Part print with two shaded views. Sizes in mm from the minimum x, y, z corner. Round coordinates to 2 decimals unless told otherwise and drop trailing zeros. Write each loop counter-clockwise with the first axis right and the second up, starting at its lowest first coordinate (ties: lowest second). Pieces come first, ordered by that corner, then holes. Notation, with made-up numbers: M -22.75,13.25 L -6.75,13.25 A10 ccw -6.75,31.25 Z; hole C 85.25,75 d1. An arc over 180 degrees is marked long. One line per question, with ' | ' between items. Start each with the question number.
1) Mould opens along Y. For the marked faces 1, 2 and 3 say: pulls with the +Y half, pulls with the -Y half, needs draft (parallel to the pull), parting line crosses it, or undercut.
2) Saw through at B-B (z = 50.8). List the corners of the cut face in (x, y).
3) Saw through at A-A (x = 24.13). List the corners of the cut face in (y, z), plus the area to 3 significant figures.
4) Wall check: probe 1 along X at (y, z) = (24, 64); probe 2 along X at (y, z) = (25, 81). Give the ranges that are in metal, low to high. Write a range as [from, to].
5) Saw through at C-C (y = 30.5). List the corners of the cut face in (x, z), plus the area to 3 significant figures.
6) Saw through at D-D (x = 45). List the corners of the cut face in (y, z), plus the area to 3 significant figures.
7) Drop flat-ended pins along their axis: pin 1 Ø23 at (x, y) = (24.13, 24.13) entering from -Z; pin 2 Ø10 at (y, z) = (38.5, 13.5) entering from +X; pin 3 Ø5 at (y, z) = (32.5, 26.5) entering from +X; pin 4 Ø1 at (x, z) = (14.5, 49) entering from +Y. Give the stop position or say it passes through.
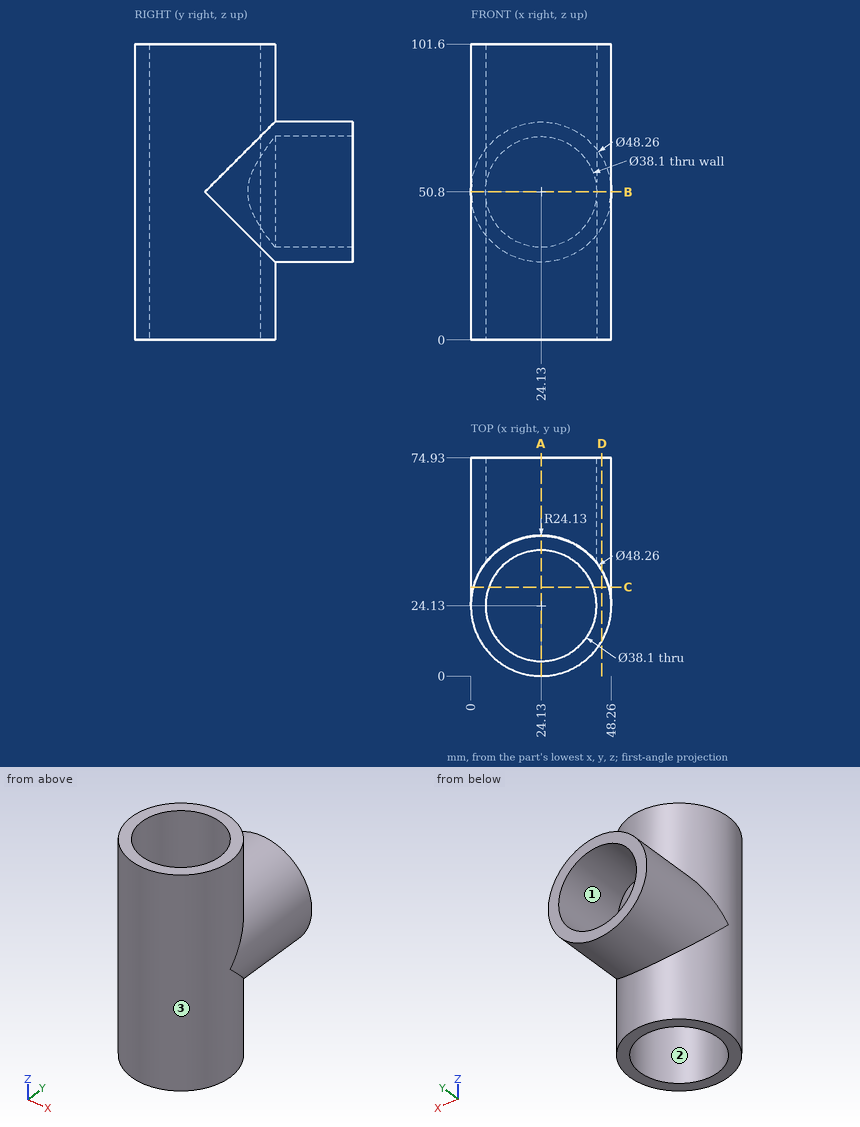
Answer key:
1) face 1: needs draft | face 2: undercut | face 3: parting line crosses it
2) outline: M 0,24.13 A24.13 ccw 48.26,24.13 L 48.26,74.93 L 43.18,74.93 L 43.18,38.94 A24.13 ccw 5.08,38.94 L 5.08,74.93 L 0,74.93 Z; hole C 24.13,24.13 d38.1
3) outline: M 0,0 L 5.08,0 L 5.08,101.6 L 0,101.6 Z; M 43.18,0 L 48.26,0 L 48.26,26.67 L 74.93,26.67 L 74.93,31.75 L 48.26,31.75 L 48.26,69.85 L 74.93,69.85 L 74.93,74.93 L 48.26,74.93 L 48.26,101.6 L 43.18,101.6 Z | area: 1,300 mm2
4) probe 1: x = [0, 5.08], [43.18, 48.26] | probe 2: x = [0.02, 5.1], [43.16, 48.24]
5) outline: M 0.86,0 L 6.18,0 L 6.18,101.6 L 0.86,101.6 L 0.86,57.17 A24.13 ccw 0.86,44.43 Z; M 42.08,0 L 47.4,0 L 47.4,44.43 A24.13 ccw 47.4,57.17 L 47.4,101.6 L 42.08,101.6 Z | area: 1,100 mm2
6) outline: M 12.02,0 L 36.24,0 L 36.24,38.69 L 74.93,38.69 L 74.93,62.91 L 36.24,62.91 L 36.24,101.6 L 12.02,101.6 Z | area: 3,400 mm2
7) pin 1: passes through | pin 2: stops at x = 46.37 | pin 3: stops at x = 47.54 | pin 4: stops at y = 46.47
